from build123d import *

# Parameters (mm, degrees)
F1_DEPTH = 2.5
F4_DEPTH = 2.5
F5_R     = 2.25
F6_DEPTH = 2.5


with BuildPart() as f1:
    # F0 (on Front) → F1 (new body)
    with BuildSketch(Plane.XZ):
        Polygon((0, 0), (70, 0), (82, 0), (82, 2), (79, 4.5), (73, 4.5), (70, 1), (65, 4.5), (60, 1), (55, 4.5), (50, 1), (45, 4.5), (40, 1), (35, 4.5), (30, 1), (25, 4.5), (20, 1), (15, 4.5), (10, 1), (5, 4.5), (0, 1), (-3, 4.5), (-9, 4.5), (-12, 2), (-12, 0), align=None)
    extrude(amount=F1_DEPTH)

    # F2: F1 across plane


with BuildPart() as f1_1:
    add(f1.part)
    add(f1.part.mirror(Plane.XY))

    # F3 (on face) → F4 (cut, through all)
    with BuildSketch(Plane.XZ.offset(2.5)):
        Polygon((5, 3), (0.75, 0), (5, -3), (9.25, 0), align=None)
        Polygon((25, 3), (20.75, 0), (25, -3), (29.25, 0), align=None)
        Polygon((35, 3), (30.75, 0), (35, -3), (39.25, 0), align=None)
        Polygon((45, 3), (40.75, 0), (45, -3), (49.25, 0), align=None)
        Polygon((55, 3), (50.75, 0), (55, -3), (59.25, 0), align=None)
        Polygon((65, 3), (60.75, 0), (65, -3), (69.25, 0), align=None)
        Polygon((15, 3), (10.75, 0), (15, -3), (19.25, 0), align=None)
    extrude(amount=-F4_DEPTH, mode=Mode.SUBTRACT)

    # F5 (on face) → F6 (cut, through all)
    with BuildSketch(Plane.XZ.offset(2.5)):
        with Locations((-6, 0)):
            Circle(F5_R)
        with Locations((76, 0)):
            Circle(F5_R)
    extrude(amount=-F6_DEPTH, mode=Mode.SUBTRACT)


solid = f1_1.part
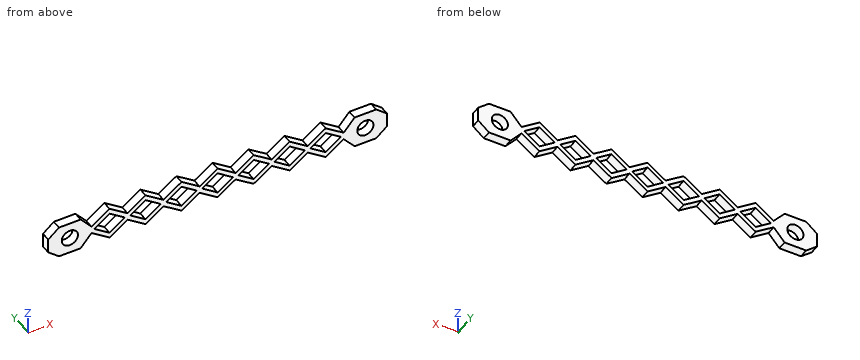
Could you check a few things on this model? Use its own coordinates, in mm. Give positions to 0.01 mm unless a question says otherwise; leave off trailing zeros. Loops run counter-clockwise (first coordinate to the right, second up) from the corner with the lowest first, then second, coordinate; pieces in that order, holes last. Notation, with made-up numbers: M 67.5,60.5 L 77.5,60.5 A19 cw 77.5,76.5 Z; hole C 28,44 d6. An arc over 180 degrees is marked long. Answer as a JSON object with one key per item and string values.
Q1. Suppose I cut it at A-A, the plane x = -6. List the corners of the cut face in (y, z) for me.
Values found:
{"outline": "M -2.5,-4.5 L 0,-4.5 L 0,-2.25 L -2.5,-2.25 Z; M -2.5,2.25 L 0,2.25 L 0,4.5 L -2.5,4.5 Z"}
Q2. Suppose I cut it at B-B, the plane y = -0.45. State how many separate pieces and enclosed holes the cut face has, plus the area to 3 significant figures.
Values found:
{"separate pieces": "1", "enclosed holes": "9", "area": "355 mm²"}
Q3. For P1, Ø4, axis at x = 76, z = 0, coming from the +Y side, with a flat end and sliding along its axis, tell me the tip position at first contact or that it passes through.
Values found:
{"P1": "passes through"}
Q4. If I drill on probe 1 along Z at (x, y) = (76, -0.6); probe 2 along Z at (x, y) = (62.5, -0.3); probe 3 along Z at (x, y) = (-2.5, -0.8), over which ranges is the centre line in solid material (lowest first)? Write a range as [from, to].
Values found:
{"probe 1": "z = [-4.5, -2.25], [2.25, 4.5]", "probe 2": "z = [-2.75, -1.24], [1.24, 2.75]", "probe 3": "z = [-3.92, 3.92]"}
